```python
from build123d import *

# Parameters (mm, degrees)
SZKIC1_R                    = 15
DODANIE_WYCI_GNI_CIE1_DEPTH = 15
DODANIE_WYCI_GNI_CIE1_TAPER = 8
SZKIC1_3_R                  = 11
DODANIE_WYCI_GNI_CIE2_DEPTH = 16
DODANIE_WYCI_GNI_CIE3_START = -16
SZKIC1_4_W                  = 30
SZKIC1_4_H                  = 38
DODANIE_WYCI_GNI_CIE3_DEPTH = 15
DODANIE_WYCI_GNI_CIE4_START = -31
SZKIC1_5_W                  = 11
SZKIC1_5_H                  = 39
DODANIE_WYCI_GNI_CIE4_DEPTH = 18
ZAOKR_GLENIE1_R             = 4


with BuildPart() as part:
    # Szkic1 → Dodanie-wyci_gni_cie1 (new body)
    with BuildSketch(Plane(origin=(0, 0, 0), x_dir=(1, 0, 0), z_dir=(0, 1, 0))):
        Circle(SZKIC1_R)
    extrude(amount=DODANIE_WYCI_GNI_CIE1_DEPTH, taper=DODANIE_WYCI_GNI_CIE1_TAPER)

    # Szkic1_3 → Dodanie-wyci_gni_cie2 (add)
    with BuildSketch(Plane(origin=(0, 0, 0), x_dir=(1, 0, 0), z_dir=(0, 1, 0))):
        Circle(SZKIC1_3_R)
    extrude(amount=-DODANIE_WYCI_GNI_CIE2_DEPTH)

    # Szkic1_4 → Dodanie-wyci_gni_cie3 (add)
    with BuildSketch(Plane(origin=(0, 0, 0), x_dir=(1, 0, 0), z_dir=(0, 1, 0)).offset(DODANIE_WYCI_GNI_CIE3_START)):
        Rectangle(SZKIC1_4_W, SZKIC1_4_H)
    extrude(amount=-DODANIE_WYCI_GNI_CIE3_DEPTH)

    # Szkic1_5 → Dodanie-wyci_gni_cie4 (add)
    with BuildSketch(Plane(origin=(0, 0, 0), x_dir=(1, 0, 0), z_dir=(0, 1, 0)).offset(DODANIE_WYCI_GNI_CIE4_START)):
        Rectangle(SZKIC1_5_W, SZKIC1_5_H)
    extrude(amount=-DODANIE_WYCI_GNI_CIE4_DEPTH)

    # Szkic2 → Obr_t1 (revolve)
    with BuildSketch(Plane(origin=(0, 0, 0), x_dir=(0, 0, -1), z_dir=(1, 0, 0))):
        Polygon((0, 15), (0, 25), (11, 25), (18.5, 22), (18.5, 16), (12, 16), (12, 15), align=None)
    revolve(axis=Axis((0, 34.075059211, 0), (0, -1, 0)))

    # Zaokr_glenie1
    zaokr_glenie1_edges = [part.edges().sort_by_distance(p)[0] for p in [
        (0, -16, -19),
        (0, -16, 19),
    ]]
    fillet(zaokr_glenie1_edges, radius=ZAOKR_GLENIE1_R)


solid = part.part
```
Work out the finished part from the listing and answer in its coordinate system (mm). A direction names the side the tool comes from. Give positions to 0.01 mm unless a question says otherwise; leave off trailing zeros. Order: outer loops, then holes, each group sorted by start corner. A loop starts at its lowest first (then second) coordinate and runs counter-clockwise, first axis right, second up. Notation, with made-up numbers: M -38.5,38.25 L 4.5,38.25 A20 cw 4.5,45.25 Z; hole C -15.75,-23.75 d10. An arc over 180 degrees is marked long. Return JSON: item names as keys, results as strings.
1) Section A-A, the plane x = 0 is taken. Write down the section's boundary in (y, z).
Resolved:
{"outline": "M -49,-19.5 L -31,-19.5 L -31,-19 L -20,-19 A4 ccw -16,-15 L -16,-11 L 0,-11 L 0,-15 L 15,-12.89 L 15,-12 L 16,-12 L 16,-18.5 L 22,-18.5 L 25,-11 L 25,11 L 22,18.5 L 16,18.5 L 16,12 L 15,12 L 15,12.89 L 0,15 L 0,11 L -16,11 L -16,15 A4 ccw -20,19 L -31,19 L -31,19.5 L -49,19.5 Z"}
2) Each of these flat-tipped pins is pushed along its axis until it touches: pin 1 (1 mm diameter, centred on y = -7, z = -1, fed in from +X); pin 2 (3.5 mm diameter, centred on x = 0.5, y = -28, fed in from +Z); pin 3 (6 mm diameter, centred on y = 3.5, z = 3, fed in from +X). Where does it stop, or does it pass through?
Resolved:
{"pin 1": "x = 10.99", "pin 2": "z = 19", "pin 3": "x = 14.8"}
3) Section D-D, the plane y = 10.5 is taken. Write down the section's boundary in (x, z), plus the area to 3 significant figures.
Resolved:
{"outline": "C 0,0 d27.05", "area": "575 mm^2"}
4) For a pull along Y with two mould halves and no side action, classify faces 5 (the flat face through (0, -25, 19)), 6 (the conical face through (-11.2, 24.81, 2.49)), 7 (the cylindrical face through (-2.38, -7.89, 10.74)), 8 (the flat face through (0, -49, 0)) as +Y half, -Y half, draft (parallel to the pull), parting line (faces both ways), or undercut.
Resolved:
{"face 5": "draft", "face 6": "+Y half", "face 7": "undercut", "face 8": "-Y half"}
5) Section C-C, the plane y = -41 is taken. Write down the section's boundary in (x, z).
Resolved:
{"outline": "M -5.5,-19.5 L 5.5,-19.5 L 5.5,19.5 L -5.5,19.5 Z"}
6) Section B-B, the plane y = -4.5 is taken. Write down the section's boundary in (x, z), plus the area to 3 significant figures.
Resolved:
{"outline": "C 0,0 d22", "area": "380 mm^2"}
7) Straight lines are drawn through the part: line 1 along X through (y, z) = (-40.5, -1.5); line 2 along X through (y, z) = (-19, 12); line 3 along Z through (x, y) = (-9.5, -20). For each, find the intervals that lie inside material, in ascending order. Write a range as [from, to].
Resolved:
{"line 1": "[-5.5, 5.5]", "line 2": "[-15, 15]", "line 3": "[-19, 19]"}
8) A tool of negligible diameter and unlimited length cuts with its end or side. For faces 1 (the flat face through (-7, -16, -10)), 2 (the cylindrical face through (0.21, -17.203, -17.859)), 3 (the flat face through (10, -31, 0)), 4 (the flat face through (-10, -31, 0)), from which of +Z, -Z, +X, -X, +Y, -Y can it reach the whole face along a straight path? Write none if from no direction.
Resolved:
{"face 1": "none", "face 2": "-Z, +X, -X", "face 3": "+Z, -Z, +X, -Y", "face 4": "+Z, -Z, -X, -Y"}
